Answer from the drawing. Dimensions are ordinates in mm from the lowest x, y and z of the part. A direction names the side the tool comes from. Round coordinates to 2 decimals unless told otherwise and drop trailing zeros. Loops run counter-clockwise (first coordinate to the right, second up) from the corner with the lowest first, then second, coordinate; pieces in that order, holes last.
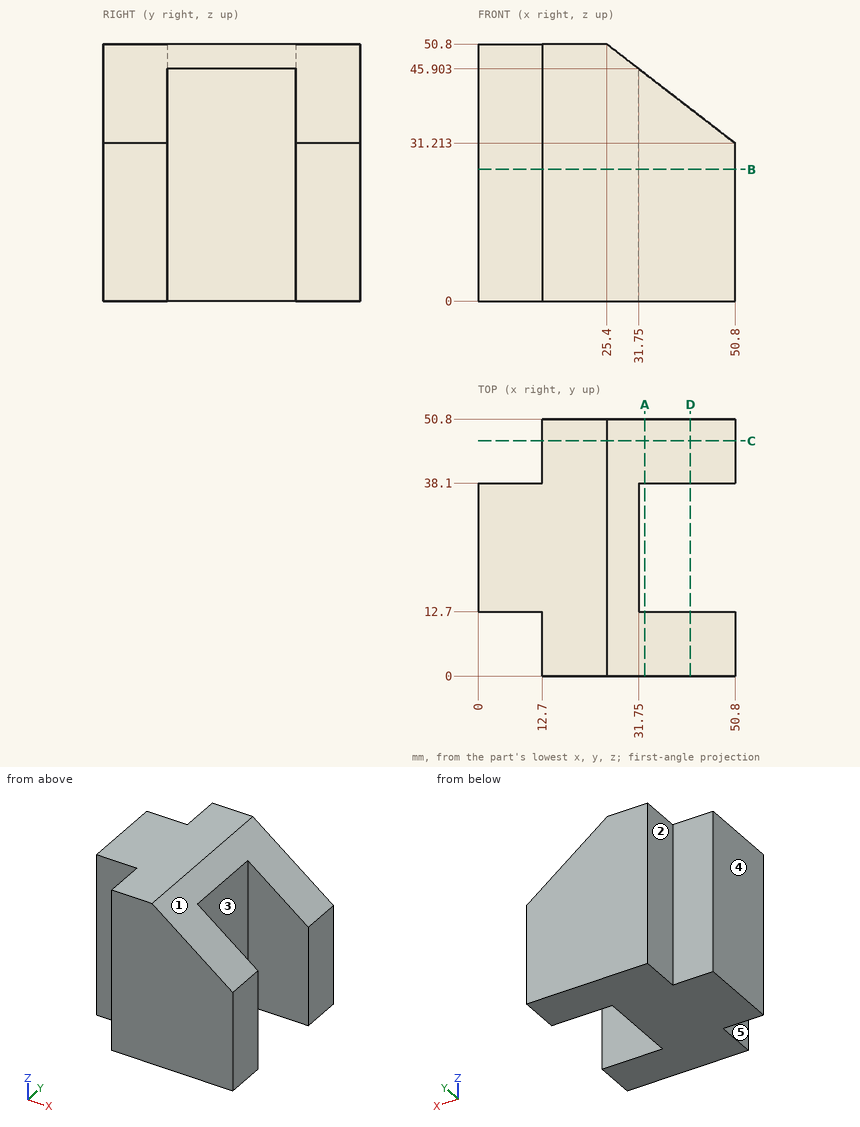
1. Find section C-C (y = 46.5). Write down the section's boundary in (x, z), then the cut area to 3 significant figures.
Answer key:
outline: (12.7, 0) - (50.8, 0) - (50.8, 31.21) - (25.4, 50.8) - (12.7, 50.8) - close
area: 1,690 mm2
2. Find section A-A (x = 33). Write down the section's boundary in (y, z), then the cut area to 3 significant figures.
Answer key:
outline: (0, 0) - (12.7, 0) - (12.7, 44.94) - (0, 44.94) - close; (38.1, 0) - (50.8, 0) - (50.8, 44.94) - (38.1, 44.94) - close
area: 1,140 mm2
3. Consider probe 1 along Y at (x, z) = (49.5, 26.5); probe 2 along X at (y, z) = (4.5, 19.5); probe 3 along X at (y, z) = (27, 9). Determine where each line is inside the solid, lowest interval first.
Answer key:
probe 1: y = 0 to 12.7, 38.1 to 50.8
probe 2: x = 12.7 to 50.8
probe 3: x = 0 to 31.75
4. Given pin 1 (7.5 mm diameter, centred on y = 23.5, z = 17.5, fed in from +X); pin 2 (6.5 mm diameter, centred on y = 42, z = 36, fed in from -X); pin 3 (6.5 mm diameter, centred on x = 7, z = 21, fed in from +Y), each flat-ended and moving along its own axis, determine where each tip first touches the part or whether it passes through.
Answer key:
pin 1: stops at x = 31.75
pin 2: stops at x = 12.7
pin 3: stops at y = 38.1
5. Find section D-D (x = 42). Write down the section's boundary in (y, z).
Answer key:
outline: (0, 0) - (12.7, 0) - (12.7, 38) - (0, 38) - close; (38.1, 0) - (50.8, 0) - (50.8, 38) - (38.1, 38) - close
6. Find section B-B (z = 26). Write down the section's boundary in (x, y), then the cut area to 3 significant figures.
Answer key:
outline: (0, 12.7) - (12.7, 12.7) - (12.7, 0) - (50.8, 0) - (50.8, 12.7) - (31.75, 12.7) - (31.75, 38.1) - (50.8, 38.1) - (50.8, 50.8) - (12.7, 50.8) - (12.7, 38.1) - (0, 38.1) - close
area: 1,770 mm2
7. Which of the six approach directions +Z, -Z, +X, -X, +Y, -Y give full straight-line access (tool end or side, diameter ignored) to the marked faces 1, 2, 3, 4 and 5?
Answer key:
face 1: +Z, +X, +Y, -Y
face 2: +Z, -Z, -X, +Y
face 3: +Z, -Z, +X
face 4: +Z, -Z, -X, +Y, -Y
face 5: +Z, -Z, -X, -Y
